Here's the drawing with two shaded views (mm, measured from the low corner). I have some questions. Coordinates: 2 decimals unless noted, no trailing zeros. Write each loop counter-clockwise with the first axis right and the second up, starting at its lowest first coordinate (ties: lowest second). Pieces come first, ordered by that corner, then holes.
Item 1: I want a section at A-A on z = 147. Please give me the cut outline in (x, y), then the cut area to 3 significant figures.
Item 2: For P1, Ø1.5, axis at y = 2, z = 149, coming from the -X side; P2, Ø0.9, axis at y = 2, z = 152, coming from the +X side; P3, Ø0.9, axis at x = 172.5, y = 1, coming from the -Z side, each with a flat end and sliding along its axis, tell me the tip position at first contact or that it passes through.
Item 3: I want a section at B-B on y = 1.4. Please give me the cut outline in (x, z).
Item 4: If I drill on probe 1 along X at (y, z) = (1.45, 158); probe 2 along Z at (x, y) = (152, 0.3); probe 3 along X at (y, z) = (0.9, 15), over which ranges is the centre line in solid material (lowest first)?
Item 5: I want a section at C-C on x = 41.5. Please give me the cut outline in (y, z).
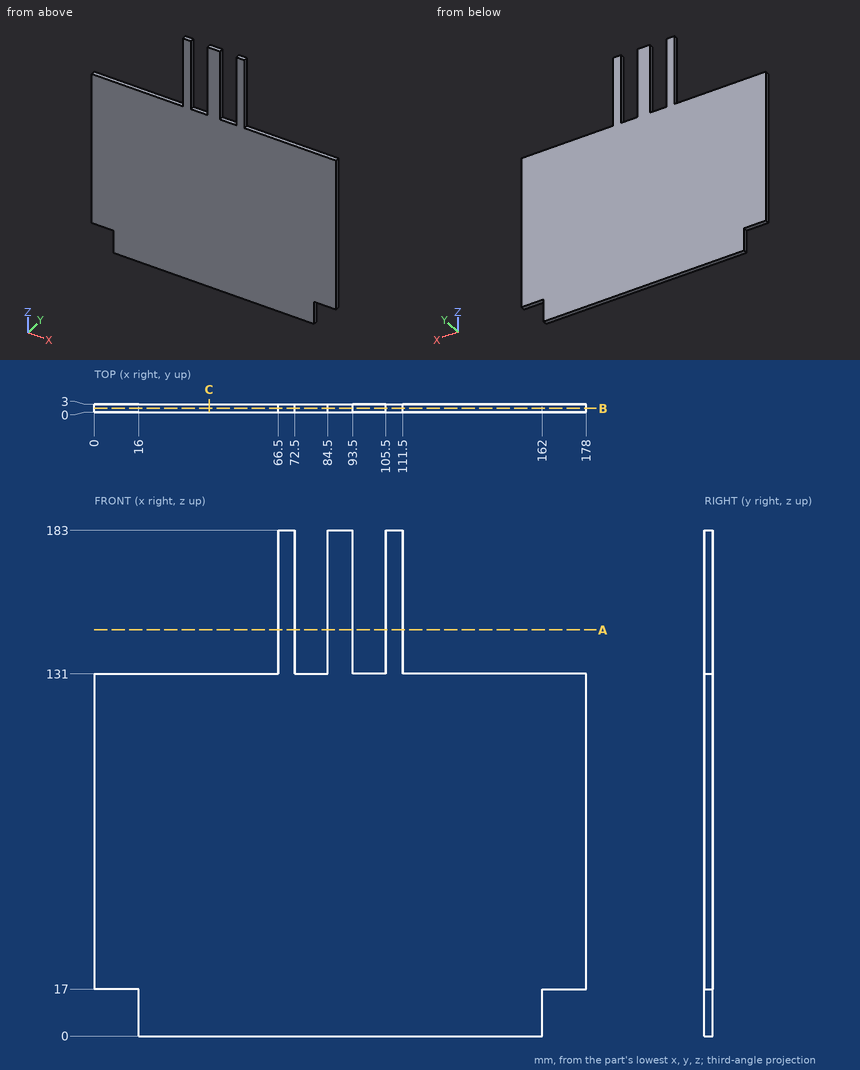
Response values:
1. outline: (66.5, 0) - (72.5, 0) - (72.5, 3) - (66.5, 3) - close; (84.5, 0) - (93.5, 0) - (93.5, 3) - (84.5, 3) - close; (105.5, 0) - (111.5, 0) - (111.5, 3) - (105.5, 3) - close
1. area: 63.0 mm2
2. P1: stops at x = 66.5
2. P2: stops at x = 111.5
2. P3: stops at z = 17
3. outline: (0, 17) - (16, 17) - (16, 0) - (162, 0) - (162, 17) - (178, 17) - (178, 131) - (111.5, 131) - (111.5, 183) - (105.5, 183) - (105.5, 131) - (93.5, 131) - (93.5, 183) - (84.5, 183) - (84.5, 131) - (72.5, 131) - (72.5, 183) - (66.5, 183) - (66.5, 131) - (0, 131) - close
4. probe 1: x = 66.5 to 72.5, 84.5 to 93.5, 105.5 to 111.5
4. probe 2: z = 0 to 131
4. probe 3: x = 16 to 162
5. outline: (0, 0) - (3, 0) - (3, 131) - (0, 131) - close
